Part model, mm, in its own coordinate system. Face numbers are marked on the shaded views. Round coordinates to 2 decimals unless told otherwise and drop trailing zeros. Order: outer loops, then holes, each group sorted by start corner. A loop starts at its lowest first (then second) coordinate and runs counter-clockwise, first axis right, second up. Notation, with made-up numbers: (76.25, 24.25) - (120.25, 24.25) arc R9 cw to (120.25, 36.25) - close; hole circle Ø10 at (60, 67.25). An arc over 180 degrees is marked (long way). Answer as a JSON object with one key per item and string values.
```python
from build123d import *

# Parameters (mm, degrees)
F0_W     = 50.8
F0_H     = 25.4
F0_W_2   = 44.45
F0_H_2   = 19.05
F1_DEPTH = 1.058333
F3_DEPTH = 25.4


with BuildPart() as f1:
    # F0 (on Front) → F1 (new body)
    with BuildSketch(Plane.XZ):
        Rectangle(F0_W, F0_H)
        Rectangle(F0_W_2, F0_H_2, mode=Mode.SUBTRACT)
    extrude(amount=F1_DEPTH)

    # F2 (on Right) → F3 (join, symmetric)
    with BuildSketch(Plane.YZ):
        Polygon((0, 10.541), (0, 9.525), (1.016, 9.525), (1.016, 9.779), (0.625132, 9.779), (0.625132, 10.287), (1.016, 10.287), (1.016, 10.541), align=None)
        Polygon((0, -9.525007), (0, -10.541007), (1.016, -10.541007), (1.016, -10.287007), (0.625132, -10.287007), (0.625132, -9.779007), (1.016, -9.779007), (1.016, -9.525007), align=None)
    extrude(amount=F3_DEPTH, both=True)


solid = f1.part
```
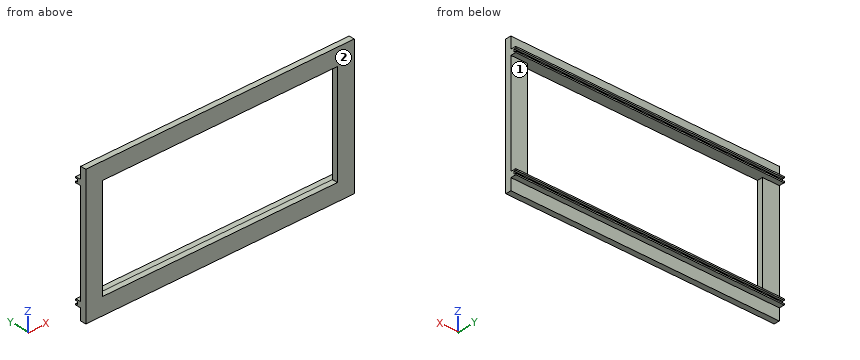
Item 1: Drop flat-ended pins along their axis: P1, Ø12, axis at x = -11.5, z = -6.5, coming from the +Y side; P2, Ø10, axis at x = -13.5, z = 4, coming from the +Y side; P3, Ø0.5, axis at x = 7, y = 0.5, coming from the -Z side; P4, Ø1.7, axis at x = 1.5, z = 11.5, coming from the +Y side. Give the stop position or say it passes through.
Taken from the geometry:
{"P1": "y = 1.02", "P2": "through", "P3": "z = -10.54", "P4": "y = 0"}
Item 2: Cut at D-D (z = -11). Write the cut outline in (x, y), plus the area to 3 significant figures.
Taken from the geometry:
{"outline": "(-25.4, -1.06) - (25.4, -1.06) - (25.4, 0) - (-25.4, 0) - close", "area": "53.8 mm2"}
Item 3: Two-plate mould, pull along Z, no slides. Class the marked faces 1 and 2: pulls with the +Z half, pulls with the -Z half, needs draft (parallel to the pull), parting line crosses it, or undercut.
Taken from the geometry:
{"face 1": "undercut", "face 2": "needs draft"}
Item 4: Cut at C-C (y = -0.45). Write the cut outline in (x, z) (3 decimals).
Taken from the geometry:
{"outline": "(-25.4, -12.7) - (25.4, -12.7) - (25.4, 12.7) - (-25.4, 12.7) - close; hole (-22.225, -9.525) - (22.225, -9.525) - (22.225, 9.525) - (-22.225, 9.525) - close"}
Item 5: Cut at A-A (z = -4.5). Write the cut outline in (x, y) (3 decimals), plus the area to 3 significant figures.
Taken from the geometry:
{"outline": "(-25.4, -1.058) - (-22.225, -1.058) - (-22.225, 0) - (-25.4, 0) - close; (22.225, -1.058) - (25.4, -1.058) - (25.4, 0) - (22.225, 0) - close", "area": "6.72 mm2"}
Item 6: Probe L1, parallel to Z at x = -6, y = 0.9 (3 decimals); L2, parallel to Z at x = -19, y = -0.2 (3 decimals); L3, parallel to X at y = -0.8, z = -0.75 (3 decimals). List the from-to ranges inside material, lowest first. Write a range as from..to.
Taken from the geometry:
{"L1": "-10.541..-10.287, -9.779..-9.525, 9.525..9.779, 10.287..10.541", "L2": "-12.7..-9.525, 9.525..12.7", "L3": "-25.4..-22.225, 22.225..25.4"}
